Verification items for the finished model (mm, model axes). Face numbers are marked on the shaded views. A direction names the side the tool comes from. Give positions to 0.01 mm unless a question says otherwise; leave off trailing zeros. Loops run counter-clockwise (first coordinate to the right, second up) from the corner with the lowest first, then second, coordinate; pieces in that order, holes last. Notation, with made-up numbers: M 40,66 L 61,66 A19 ccw 61,91 Z; hole C -12.75,69 d2. An arc over 180 degrees is marked long. Answer in a Markdown table with one row per item.
```python
from build123d import *

# Parameters (mm, degrees)
EXTRUDE_1_DEPTH     = 15
CUT_EXTRUDE_2_DEPTH = 6
EXTRUDE_2_DEPTH     = 2


with BuildPart() as part:
    # Эскиз1 → Бобышка-Вытянуть1 (new body, symmetric)
    with BuildSketch(Plane.XY):
        Polygon((0, 37), (0, 0), (35, 0), (35, 5), (5, 5), (5, 37), align=None)
    extrude(amount=EXTRUDE_1_DEPTH, both=True)

    # Эскиз5 → Вырез-Вытянуть2 (cut, through all)
    with BuildSketch(Plane(origin=(0, 5, 0), x_dir=(1, 0, 0), z_dir=(0, 1, 0))):
        with BuildLine():
            Line((35, 15), (20, 15))
            ThreePointArc((20, 15), (30.606601718, 10.606601718), (35, 0))
            Line((35, 0), (35, 15))
        make_face()
        with BuildLine():
            Line((35, -15), (35, 0))
            ThreePointArc((35, 0), (30.606601718, -10.606601718), (20, -15))
            Line((20, -15), (35, -15))
        make_face()
    extrude(amount=-CUT_EXTRUDE_2_DEPTH, mode=Mode.SUBTRACT)

    # Эскиз2 → Бобышка-Вытянуть2 (add)
    with BuildSketch(Plane.XY.offset(15)):
        Polygon((5, 33), (20, 5), (5, 5), align=None)
    extrude_2 = extrude(amount=-EXTRUDE_2_DEPTH)

    # Зеркальное отражение2: Бобышка-Вытянуть2 across plane
    add(extrude_2.mirror(Plane.XY))

    # Эскиз8 → Зенковка для винта с полупотайной головкой M61 (revolve, cut)
    with BuildSketch(Plane(origin=(20, 5, 0), x_dir=(0, 0, 1), z_dir=(1, 0, 0))):
        Polygon((0, 0), (0, 11.202797012), (3.25, 9.25), (3.25, 3.05), (6.3, 0), align=None)
    hole_wizard_m61 = revolve(axis=Axis((20, 11.35, 0), (0, -1, 0)), mode=Mode.SUBTRACT)

    # Зеркальное отражение3: Зенковка для винта с полупотайной головкой M61 across plane
    add(hole_wizard_m61.mirror(Plane(origin=(0, 0, 0), x_dir=(0, 0, 1), z_dir=(-0.707106781, 0.707106781, 0))), mode=Mode.SUBTRACT)


solid = part.part
```
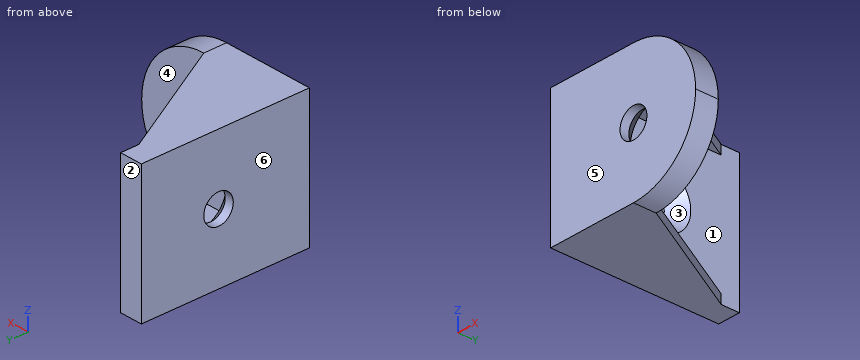
Item 1: Release check for a two-part mould opening along Y. For the marked faces 3, 4, 5 and 6 record: released by +Y, released by -Y, zero draft, split by the parting line, or undercut.
Reported:
| item | result |
|---|---|
| face 3 | undercut |
| face 4 | released by +Y |
| face 5 | released by -Y |
| face 6 | zero draft |
Item 2: Go/stop test with flat-tipped pins: pin 1 (15 mm diameter, centred on x = 13.5, z = -4.5, fed in from +Y); pin 2 (9 mm diameter, centred on y = 25.5, z = 6.5, fed in from +X); pin 3 (7.5 mm diameter, centred on x = 20, z = 0, fed in from +Y). Record where each tip stops, or that it passes through.
Reported:
| item | result |
|---|---|
| pin 1 | stops at y = 5 |
| pin 2 | stops at x = 5 |
| pin 3 | stops at y = 2.45 |
Item 3: Sectioned sample at C-C (z = 10.25). Record the cut outline in (x, y).
Reported:
| item | result |
|---|---|
| outline | M 0,0 L 30.95,0 L 30.95,5 L 5,5 L 5,37 L 0,37 Z |
Item 4: Tool access check on the marked faces 1 and 2. Record the directions out of +Z, -Z, +X, -X, +Y, -Y that give a thin tool (end or side, any length) a straight path to the whole face; none if there is none.
Reported:
| item | result |
|---|---|
| face 1 | +X, +Y |
| face 2 | +Z, -Z, +X, -X, +Y |
Item 5: Sectioned sample at B-B (y = 20). Record the cut outline in (x, z).
Reported:
| item | result |
|---|---|
| outline | M 0,-15 L 11.96,-15 L 11.96,-13 L 5,-13 L 5,-6.3 L 1.95,-3.25 L 0,-3.25 Z; M 0,3.25 L 1.95,3.25 L 5,6.3 L 5,13 L 11.96,13 L 11.96,15 L 0,15 Z |
Item 6: Sectioned sample at D-D (y = 32). Record the cut outline in (x, z).
Reported:
| item | result |
|---|---|
| outline | M 0,-15 L 5.54,-15 L 5.54,-13 L 5,-13 L 5,13 L 5.54,13 L 5.54,15 L 0,15 Z |
Item 7: Scan lines: L1, parallel to Z at x = 8.5, y = 22; L2, parallel to Z at x = 20, y = 1.3; L3, parallel to Y at x = 0.5, z = 0. Record each from-to range of solid material in increasing order. Write a range as [from, to].
Reported:
| item | result |
|---|---|
| L1 | z = [-15, -13], [13, 15] |
| L2 | z = [-15, -3.25], [3.25, 15] |
| L3 | y = [0, 16.75], [23.25, 37] |
Item 8: Sectioned sample at A-A (y = 3.5). Record the cut outline in (x, z), and give its area (3 significant figures).
Reported:
| item | result |
|---|---|
| outline | M 0,-15 L 20,-15 A15 ccw 20,15 L 0,15 Z; hole C 20,0 d9.6 |
| area | 881 mm^2 |
